Job drawing, mm, ordinate dimensions from the low corner. One solid piece. Give positions to 0.01 mm unless a question says otherwise; leave off trailing zeros. Write each loop counter-clockwise with the first axis right and the second up, starting at its lowest first coordinate (ties: lowest second). Pieces come first, ordered by that corner, then holes. Notation, with made-up numbers: (21.5, 61) -> (76.5, 61) arc R30 ccw to (76.5, 83) -> close; hole circle Ø1 at (-18, 10). An arc over 180 degrees is marked (long way). Put each result on its own line as item: value. Start each with the question number.
Item 1: Slice it at C-C, the plane x = 22. List the corners of the cut face in (y, z).
Item 2: Drill centre lines: line 1 along Z through (x, y) = (6, 7); line 2 along X through (y, z) = (2.25, 7.5); line 3 along X through (y, z) = (6.75, 45). Where is each one in solid material? Low to high.
Item 3: Flat gauge pin, fed straight in: pin 1 Ø2 at (x, y) = (8, 5) entering from -Z. Where does the tip first touch, or does it go through?
Item 4: Two-plate mould, pull along X, no slides. Class the marked faces 1, 2 and 3: pulls with the +X half, pulls with the -X half, needs draft (parallel to the pull), parting line crosses it, or undercut.
Item 5: Slice it at A-A, the plane y = 4.25. List the corners of the cut face in (x, z), plus the area to 3 significant figures.
Item 6: Slice it at B-B, the plane z = 5. List the corners of the cut face in (x, y).
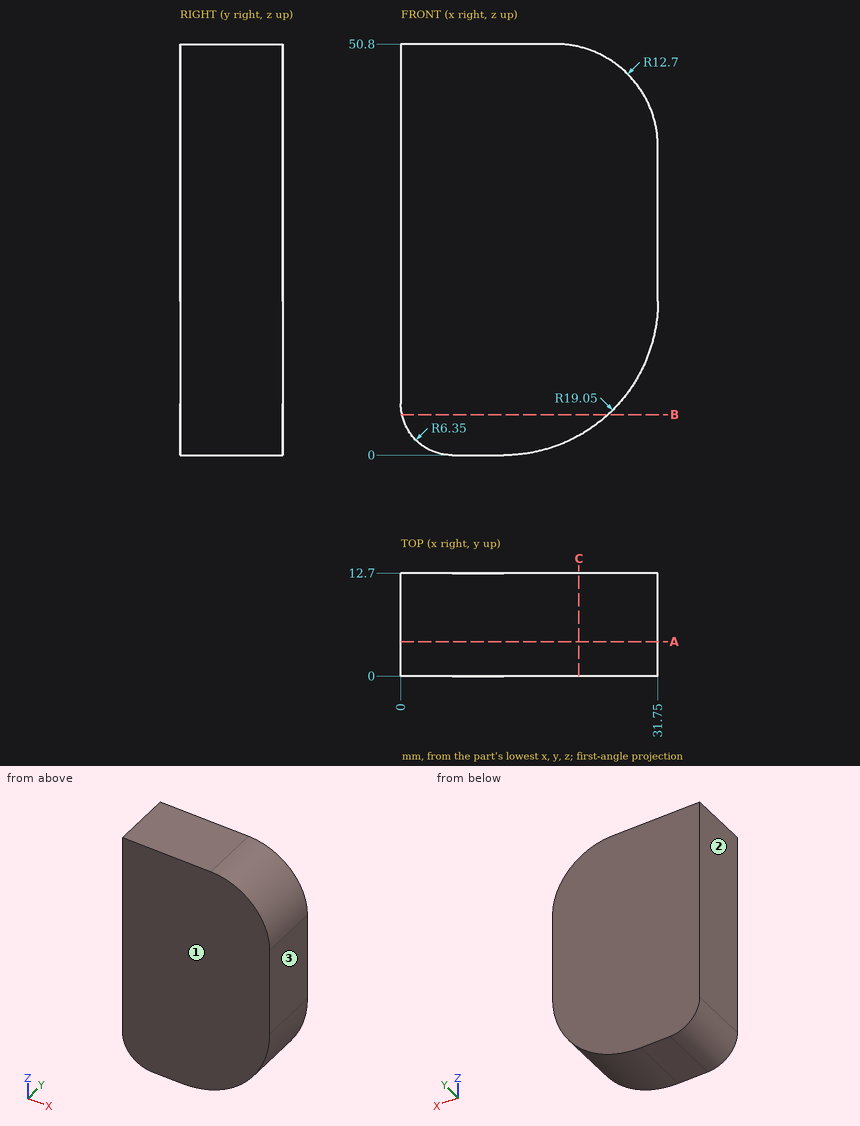
Values follow:
1. outline: (0, 2.42) -> (12.7, 2.42) -> (12.7, 50.45) -> (0, 50.45) -> close
2. line 1: 0.01 to 50.8
2. line 2: 0 to 27.85
2. line 3: 0 to 29.71
3. pin 1: z = 0
4. face 1: needs draft
4. face 2: pulls with the -X half
4. face 3: pulls with the +X half
5. outline: (0, 6.35) arc R6.35 ccw to (6.35, 0) -> (12.7, 0) arc R19.05 ccw to (31.75, 19.05) -> (31.75, 38.1) arc R12.7 ccw to (19.05, 50.8) -> (0, 50.8) -> close
5. area: 1,490 mm2
6. outline: (0.15, 0) -> (25.56, 0) -> (25.56, 12.7) -> (0.15, 12.7) -> close
